Input: part model. Units: mm. Frame: model coordinates. Coordinates: 2 decimals unless noted, no trailing zeros. Order: outer loops, then holes, each group sorted by start corner. A loop starts at its lowest first (then second) coordinate and runs counter-clockwise, first axis right, second up. Notation, with made-up numbers: (-34, 86.5) -> (-13, 86.5) arc R23 ccw to (-13, 99.5) -> close; hole circle Ø6 at (-17, 72). An arc over 180 degrees is marked (long way). Use one line per item in the form item = value. Start each with the question number.
1) Ray query, line 1 along X through (y, z) = (0.9, 0); line 2 along X through (y, z) = (1.95, -3.25); line 3 along Z through (x, y) = (-7.5, 2.7). Return the intervals inside material, ascending.
2) Section query C-C on y = 2.8. Output: boundary loops of the cut face in (x, z), then the cut area to 3 significant figures.
3) Section query A-A on z = 0. Output: boundary loops of the cut face in (x, y).
4) Section query B-B on x = 0. Output: boundary loops of the cut face in (y, z), then the cut area to 3 significant figures.
5) Draft query along X for faces 1 (the flat face through (4, 0, 4)), 2 (the cylindrical face through (-1.02, 0.71, 4.59)). Return one class per face: pulls with the +X half, pulls with the -X half, needs draft (parallel to the pull), parting line crosses it, or undercut.
6) Section query D-D on y = 0.5. Output: boundary loops of the cut face in (x, z), then the cut area to 3 significant figures.
Autodesk Inventor part; units mm, degrees
ref_plane "YZ Plane" through (0, 0, 0) normal (1, 0, 0) x (0, 1, 0)
ref_plane "XZ Plane" through (0, 0, 0) normal (0, 1, 0) x (-1, 0, 0)
ref_plane "XY Plane" through (0, 0, 0) normal (0, 0, 1) x (1, 0, 0)
sketch "Sketch1" plane through (0, 0, 0) normal (0, 0, 1) x (1, 0, 0)
  line L0 (11.9, 0) -> (11.9, 3.5) construction
  line L1 (11.9, 3.5) -> (10.5, 3.5) construction
  line L2 (0, 0) -> (0, 1.4)
  line L3 (10.5, 3.5) -> (10.5, 4) construction
  line L4 (11.9, 3.5) -> (10.5, 4)
  line L5 (0, 0) -> (10.5, 0)
  line L6 (10.5, 0) -> (11.9, 3.5)
  line L7 (10.5, 4) -> (9.46, 1.4)
  line L8 (0, 1.4) -> (9.46, 1.4)
  dimension "d0" = 11.9
  dimension "d1" = 3.5
  dimension "d2" = 1.4
  dimension "d3" = 0.5
  dimension "d4" = 1.4
revolve "Revolution1" add sketch "Sketch1" angle 360 about axis through (0, 0, 0) along (0, 1, 0)
sketch "Sketch2" plane through (0, 1.4, 0) normal (0, 1, 0) x (1, 0, 0)
  circle A0 centre (0, 0) radius 4.7
  dimension "d6" = 9.4
extrude "Extrusion1" cut sketch "Sketch2" against normal through all
fillet "Fillet1" radius 2.4 1 edges at (-10.5, 0, 0)
properties part number "TopBushingWasher" material "Aluminum"
Answers below:
q1.line_1 = -10.75 to -4.7, 4.7 to 10.75
q1.line_2 = -10.8 to -9.12, 9.12 to 10.8
q1.line_3 = -8.82 to -6.58, 6.58 to 8.82
q2.outline = circle Ø23.24 at (0, 0); hole circle Ø20.04 at (0, 0)
q2.area = 109 mm^2
q3.outline = (-11.9, 3.5) -> (-11.1, 1.51) arc R2.4 ccw to (-8.88, 0) -> (-4.7, 0) -> (-4.7, 1.4) -> (-9.46, 1.4) -> (-10.5, 4) -> close; (4.7, 0) -> (8.88, 0) arc R2.4 ccw to (11.1, 1.51) -> (11.9, 3.5) -> (10.5, 4) -> (9.46, 1.4) -> (4.7, 1.4) -> close
q4.outline = (0, -8.88) arc R2.4 ccw to (1.51, -11.1) -> (3.5, -11.9) -> (4, -10.5) -> (1.4, -9.46) -> (1.4, -4.7) -> (0, -4.7) -> close; (0, 4.7) -> (1.4, 4.7) -> (1.4, 9.46) -> (4, 10.5) -> (3.5, 11.9) -> (1.51, 11.1) arc R2.4 ccw to (0, 8.88) -> close
q4.area = 23.6 mm^2
q5.face_1 = needs draft
q5.face_2 = undercut
q6.outline = circle Ø20.68 at (0, 0); hole circle Ø9.4 at (0, 0)
q6.area = 267 mm^2
